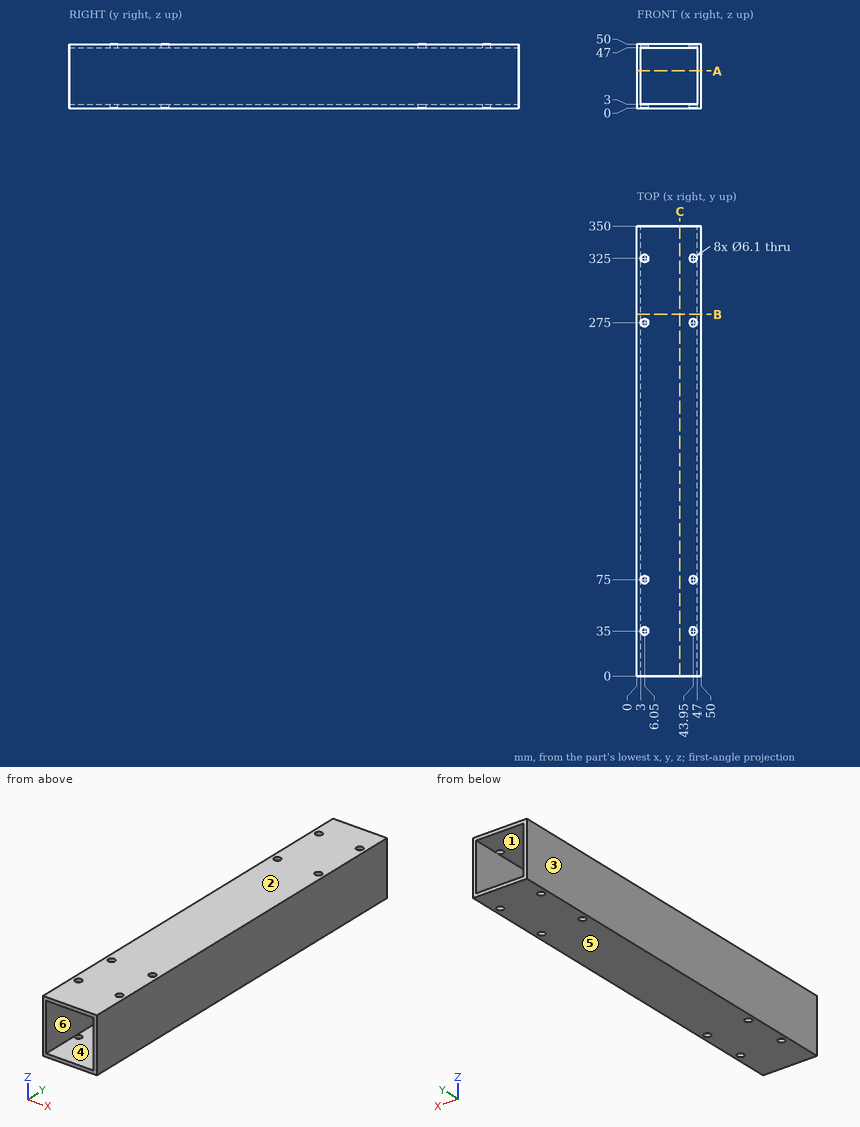
Input: dimensioned drawing with shaded views. Units: mm. Origin: part minimum x, y, z. A direction names the side the tool comes from. Give positions to 0.01 mm unless a question says otherwise; leave off trailing zeros. Order: outer loops, then holes, each group sorted by start corner. A loop starts at its lowest first (then second) coordinate and runs counter-clockwise, first axis right, second up. Notation, with made-up numbers: (18.25, 23.5) -> (48.25, 23.5) arc R23 ccw to (48.25, 52.5) -> close; hole circle Ø5 at (-5.5, -33). An arc over 180 degrees is marked (long way). Write item = value, one per line.
Item 1: Section query A-A (z = 29). Output: boundary loops of the cut face in (x, y).
Check result:
outline = (0, 0) -> (3, 0) -> (3, 350) -> (0, 350) -> close; (47, 0) -> (50, 0) -> (50, 350) -> (47, 350) -> close
Item 2: Section query B-B (y = 281.5). Output: boundary loops of the cut face in (x, z).
Check result:
outline = (0, 0) -> (50, 0) -> (50, 50) -> (0, 50) -> close; hole (3, 3) -> (47, 3) -> (47, 47) -> (3, 47) -> close
Item 3: Mould query, pull axis X, two halves, no side actions, for the marked faces 3, 4, 5 and 6. Classes: +X half, -X half, draft (parallel to the pull), parting line (faces both ways), or undercut.
Check result:
face_3 = -X half
face_4 = undercut
face_5 = draft
face_6 = undercut
Item 4: Contact query for a flat-ended pin moving along its axis: pin 1 (7 mm diameter, centred on x = 43.95, y = 275, fed in from +Z). Output: stop coordinate, or through.
Check result:
pin_1 = 50
Item 5: Ray query, probe 1 along Y at (x, z) = (6.05, 48.15); probe 2 along X at (y, z) = (325, 1.55); probe 3 along Z at (x, y) = (26, 52). Return the intervals inside material, ascending.
Check result:
probe_1 = 0 to 31.95, 38.05 to 71.95, 78.05 to 271.95, 278.05 to 321.95, 328.05 to 350
probe_2 = 0 to 3, 9.1 to 40.9, 47 to 50
probe_3 = 0 to 3, 47 to 50
Item 6: Set-up query: the marked faces 1 and 2. Return all of +Z, -Z, +X, -X, +Y, -Y with unobstructed straight access to the full face (end or side cutting, diameter ignored); none if empty.
Check result:
face_1 = +Y, -Y
face_2 = +Z, +X, -X, +Y, -Y
Item 7: Section query C-C (x = 33.5). Output: boundary loops of the cut face in (y, z), then the cut area to 3 significant figures.
Check result:
outline = (0, 0) -> (350, 0) -> (350, 3) -> (0, 3) -> close; (0, 47) -> (350, 47) -> (350, 50) -> (0, 50) -> close
area = 2,100 mm²
